Source: CAD feature listing. Evaluate the final solid. Frame: model axes, mm. A direction names the side the tool comes from. Round coordinates to 2 decimals unless told otherwise and drop trailing zeros. Order: outer loops, then holes, each group sorted by start corner. A loop starts at its lowest first (then second) coordinate and runs counter-clockwise, first axis right, second up. Notation, with made-up numbers: (69, 10) - (85, 10) arc R14 ccw to (85, 24) - close; hole circle Ø11 at (9.5, -14.5). An arc over 180 degrees is marked (long way). Use one line per item in the form item = value. Start each with the question number.
Q1. Ray query, line 1 (Z direction, x = -2, y = 3.75); line 2 (Z direction, x = -0.75, y = -2.25); line 3 (Y direction, x = 2.25, z = 0.25). Return the intervals inside material, ascending. Write a range as [from, to].
Q2. Cut plane B-B, the plane z = 3. Return the cut outline in (x, y), and give its area (3 significant figures).
Q3. Cut plane C-C, the plane z = 5. Return the cut outline in (x, y).
Q4. Draft query along X for faces 4 (the cylindrical face through (-0.7, 0.413, 4.955)), 5 (the flat face through (0, 2, 0)), 6 (the cylindrical face through (3.515, 3.012, 2.185)). Return one class per face: released by +X, released by -X, zero draft, split by the parting line, or undercut.
Q5. Pin query (flat end, axial travel): pin 1 Ø4 at (y, z) = (-7.5, 3) entering from +X; pin 2 Ø1 at (y, z) = (1.5, 4.5) entering from +X; pin 3 Ø2 at (x, y) = (2.5, -7) entering from +Z; pin 4 Ø3 at (x, z) = (2.5, 3.5) entering from +Y. Return the tip coordinate at first contact, or that it passes through.
Q6. Set-up query: faces 1 (the flat face through (-3.4, 4.8, 1.1)), 2 (the flat face through (4.054, 1.7, 0.5)), 3 (the flat face through (0, 2, 4.6)). Return all of +Z, -Z, +X, -X, +Y, -Y with unobstructed straight access to the full face (end or side cutting, diameter ignored); none if empty.
Q7. Cut plane A-A, the plane y = 1.78. Return the cut outline in (x, z), and give its area (3 significant figures).
Q8. Cut plane D-D, the plane y = -11. Return the cut outline in (x, z).
from build123d import *

# Parameters (mm, degrees)
EXTRUDE_633_DEPTH    = 0.1
SKETCH_2_W           = 8.9
SKETCH_2_H           = 8.9
EXTRUDE_2_DEPTH      = 1
SKETCH_3_R           = 4.1
EXTRUDE_3_DEPTH      = 2.5
SKETCH_4_R           = 3.719118072
EXTRUDE_4_DEPTH      = 2
SKETCH_5_R           = 4.1
EXTRUDE_5_DEPTH      = 1
EXTRUDE_5_DRAFT      = 10
SKETCH_6_R           = 1.4
CUT_EXTRUDE_1_DEPTH  = 1
FILLET_1_R           = 0.3
FILLET_2_R           = 0.3
FILLET_3_R           = 0.3
EXTRUDE_7_DEPTH      = 2.6
EXTRUDE_7_DEPTH_BACK = 0.1
CUT_EXTRUDE_4_REACH  = 21.211
CUT_EXTRUDE_5_REACH  = 23.178
SKETCH_13_W          = 2.594072948
SKETCH_13_H          = 2


with BuildPart() as part:
    # 草图1 → Extrude 633 (new body)
    with BuildSketch(Plane.XY):
        Polygon((2.653989215, -2.67), (4.053989215, -2.67), (4.053989215, 6.23), (-4.846010785, 6.23), (-4.846010785, -2.67), (-3.446010785, -2.67), (-3.446010785, -13.67), (-6.946010785, -13.67), (-6.946010785, -15.67), (6.153989215, -15.67), (6.153989215, -13.67), (2.653989215, -13.67), align=None)
    extrude(amount=EXTRUDE_633_DEPTH)

    # 草图2 → 凸台-拉伸2 (add)
    with BuildSketch(Plane.XY.offset(0.1)):
        with Locations((-0.396010785, 1.78)):
            Rectangle(SKETCH_2_W, SKETCH_2_H)
    extrude(amount=EXTRUDE_2_DEPTH)

    # 草图3 → 凸台-拉伸3 (add)
    with BuildSketch(Plane.XY.offset(1.1)):
        with Locations((-0.396010785, 1.78)):
            Circle(SKETCH_3_R)
    extrude(amount=EXTRUDE_3_DEPTH)

    # 草图4 → 凸台-拉伸4 (add)
    with BuildSketch(Plane.XY.offset(3.6)):
        with Locations((-0.396010785, 1.78)):
            Circle(SKETCH_4_R)
    extrude(amount=EXTRUDE_4_DEPTH)


with BuildPart() as extrude_5_tool:
    # 草图5 → 凸台-拉伸5 (with draft: the straight prism first)
    with BuildSketch(Plane.XY.offset(5.6)):
        with Locations((-0.396010785, 1.78)):
            Circle(SKETCH_5_R)
    extrude(amount=-EXTRUDE_5_DEPTH)
    # 凸台-拉伸5: the draft: its side faces are tilted about the plane it starts from
    extrude_5_sides = [extrude_5_tool.faces().sort_by_distance(p)[0] for p in [
        (-4.496010785, 1.78, 5.1),
    ]]
    draft(extrude_5_sides, Plane.XY.offset(5.6), EXTRUDE_5_DRAFT)


with BuildPart() as part_1:
    add(part.part)

    # 凸台-拉伸5: add extrude_5_tool
    add(extrude_5_tool.part)

    # 草图6 → 切除-拉伸1 (cut)
    with BuildSketch(Plane.XY.offset(5.6)):
        with Locations((-0.396010785, 1.78)):
            Circle(SKETCH_6_R)
    extrude(amount=-CUT_EXTRUDE_1_DEPTH, mode=Mode.SUBTRACT)

    # 圆角1
    fillet_1_edges = [part_1.edges().sort_by_distance(p)[0] for p in [
        (-4.496010785, 1.78, 3.6),
        (-4.496010785, 1.78, 5.6),
    ]]
    fillet(fillet_1_edges, radius=FILLET_1_R)

    # 圆角2
    fillet_2_edges = [part_1.edges().sort_by_distance(p)[0] for p in [
        (-4.846010785, 6.23, 0.55),
        (4.053989215, 6.23, 0.55),
        (4.053989215, -2.67, 0.55),
        (-4.846010785, -2.67, 0.55),
    ]]
    fillet(fillet_2_edges, radius=FILLET_2_R)

    # 圆角3
    fillet_3_edges = [part_1.edges().sort_by_distance(p)[0] for p in [
        (-1.796010785, 1.78, 5.6),
    ]]
    fillet(fillet_3_edges, radius=FILLET_3_R)

    # 草图11 → 凸台-拉伸7 (add, two sides: drawn at the far end of the back side and taken through both)
    with BuildSketch(Plane(origin=(0, 0, 0), x_dir=(-1, 0, 0), z_dir=(0, 0, -1)).offset(-EXTRUDE_7_DEPTH_BACK)):
        Polygon((-2.653989215, -13.67), (-6.153989215, -13.67), (-6.153989215, -15.67), (6.946010785, -15.67), (6.946010785, -13.67), (3.446010785, -13.67), (3.446010785, -2.67), (-2.653989215, -2.67), align=None)
    extrude(amount=EXTRUDE_7_DEPTH + EXTRUDE_7_DEPTH_BACK)

    # 草图12 → 切除-拉伸4 (cut, up to next)
    with BuildSketch(Plane.ZY.offset(3.446010785), mode=Mode.PRIVATE) as cut_extrude_4_sk1:
        Polygon((0, -2.67), (-2.6, -13.67), (-2.6, -2.67), align=None)
    cut_extrude_4_tool1 = extrude(cut_extrude_4_sk1.sketch, amount=-CUT_EXTRUDE_4_REACH, mode=Mode.PRIVATE) & part_1.part
    # 草图12 → 切除-拉伸4 (cut, up to next)
    with BuildSketch(Plane.ZY.offset(3.446010785), mode=Mode.PRIVATE) as cut_extrude_4_sk2:
        Polygon((0.1, -2.67), (-2.5, -13.67), (0.1, -13.67), align=None)
    cut_extrude_4_tool2 = extrude(cut_extrude_4_sk2.sketch, amount=-CUT_EXTRUDE_4_REACH, mode=Mode.PRIVATE) & part_1.part
    add(cut_extrude_4_tool1.solids().sort_by_distance((-3.446011, -6.336667, -1.733333))[0], mode=Mode.SUBTRACT)
    add(cut_extrude_4_tool2.solids().sort_by_distance((-3.446011, -10.003333, -0.766667))[0], mode=Mode.SUBTRACT)

    # 草图13 → 切除-拉伸5 (cut, up to next)
    with BuildSketch(Plane.ZY.offset(6.946010785), mode=Mode.PRIVATE) as cut_extrude_5_sk1:
        with Locations((-1.197036474, -14.67)):
            Rectangle(SKETCH_13_W, SKETCH_13_H)
    cut_extrude_5_tool1 = extrude(cut_extrude_5_sk1.sketch, amount=-CUT_EXTRUDE_5_REACH, mode=Mode.PRIVATE) & part_1.part
    add(cut_extrude_5_tool1.solids().sort_by_distance((-6.946011, -14.67, -1.197036))[0], mode=Mode.SUBTRACT)


solid = part_1.part
Completed:
q1.line_1 = [0, 5.6]
q1.line_2 = [0, 3.47], [4.6, 5.53]
q1.line_3 = [-2.67, 6.23]
q2.outline = circle Ø8.2 at (-0.4, 1.78)
q2.area = 52.8 mm2
q3.outline = circle Ø8.41 at (-0.4, 1.78); hole circle Ø2.8 at (-0.4, 1.78)
q4.face_4 = undercut
q4.face_5 = zero draft
q4.face_6 = split by the parting line
q5.pin_1 = through
q5.pin_2 = 3.88
q5.pin_3 = -0.69
q5.pin_4 = 5.63
q6.face_1 = none
q6.face_2 = +Z, -Z, +X, +Y, -Y
q6.face_3 = +Z
q7.outline = (-4.85, 0) - (4.05, 0) - (4.05, 1.1) - (3.7, 1.1) - (3.7, 3.3) arc R0.3 ccw to (3.4, 3.6) - (3.32, 3.6) - (3.32, 4.6) - (3.88, 4.6) - (3.75, 5.35) arc R0.3 ccw to (3.45, 5.6) - (1.3, 5.6) arc R0.3 ccw to (1, 5.3) - (1, 4.6) - (-1.8, 4.6) - (-1.8, 5.3) arc R0.3 ccw to (-2.1, 5.6) - (-4.24, 5.6) arc R0.3 ccw to (-4.54, 5.35) - (-4.67, 4.6) - (-4.12, 4.6) - (-4.12, 3.6) - (-4.2, 3.6) arc R0.3 ccw to (-4.5, 3.3) - (-4.5, 1.1) - (-4.85, 1.1) - close
q7.area = 43.2 mm2
q8.outline = (-3.45, -1.97) - (2.65, -1.97) - (2.65, -1.87) - (-3.45, -1.87) - close
